Can you work these out from the model? Positions are in its coordinate system, mm. A direction names the side the tool comes from. Coordinates: 2 decimals unless noted, no trailing zeros. Loops run counter-clockwise (first coordinate to the right, second up) from the corner with the lowest first, then second, coordinate; pieces in that order, holes last.
```python
from build123d import *

# Parameters (mm, degrees)
BOSS_EXTRUDE1_DEPTH      = 22
SKETCH1_3_R              = 25
BOSS_EXTRUDE2_DEPTH      = 44
BOSS_EXTRUDE2_DEPTH_BACK = 37


with BuildPart() as part:
    # Sketch1 → Boss-Extrude1 (new body)
    with BuildSketch(Plane.XY):
        Polygon((-177.8, 78.062396106), (177.8, 78.062396106), (101.6, -48.937603894), (-101.6, -48.937603894), align=None)
    extrude(amount=BOSS_EXTRUDE1_DEPTH)

    # Sketch1_3 → Boss-Extrude2 (add, two sides)
    with BuildSketch(Plane.XY) as boss_extrude2_sk:
        with Locations((177.8, 78.062396106)):
            Circle(SKETCH1_3_R)
        with Locations((101.6, -48.937603894)):
            Circle(SKETCH1_3_R)
        with Locations((-101.6, -48.937603894)):
            Circle(SKETCH1_3_R)
        with Locations((-177.8, 78.062396106)):
            Circle(SKETCH1_3_R)
    extrude(amount=BOSS_EXTRUDE2_DEPTH)
    extrude(boss_extrude2_sk.sketch, amount=-BOSS_EXTRUDE2_DEPTH_BACK)


solid = part.part
```
(1) I want a section at D-D on x = -177.8. Write out the boundary of the cut face in (y, z), then the cut area to 3 significant figures.
Check values:
outline: (53.06, -37) - (103.06, -37) - (103.06, 44) - (53.06, 44) - close
area: 4,050 mm2
(2) Which directions (+Z, -Z, +X, -X, +Y, -Y) give clear straight access to the entire face, cutting with the end or side of a thin tool? Please do faces 3 (the flat face through (-178, 78, -37)), 4 (the flat face through (-2, 78.062, 11)).
Check values:
face 3: -Z, +X, -X, +Y, -Y
face 4: +Z, -Z, +Y
(3) If I drill on probe 1 along X at (y, z) = (76, 26.5); probe 2 along X at (y, z) = (78, 40); probe 3 along Y at (x, z) = (-31.5, 14.5), over which ranges is the centre line in solid material (lowest first)?
Check values:
probe 1: x = -202.71 to -152.89, 152.89 to 202.71
probe 2: x = -202.8 to -152.8, 152.8 to 202.8
probe 3: y = -48.94 to 78.06
(4) I want a section at B-B on z = 27.5. Write out the boundary of the cut face in (x, y), then the cut area to 3 significant figures.
Check values:
outline: circle Ø50 at (-177.8, 78.06); circle Ø50 at (-101.6, -48.94); circle Ø50 at (101.6, -48.94); circle Ø50 at (177.8, 78.06)
area: 7,850 mm2
(5) If we mould it in two halves opening along X, with no side actions, what happens to faces 1 (the flat face through (-178, 78, 44)), 2 (the flat face through (1, -48.938, 11))? For each: released by +X, released by -X, zero draft, split by the parting line, or undercut.
Check values:
face 1: zero draft
face 2: undercut
(6) I want a section at C-C on y = 23. Write out the boundary of the cut face in (x, z), then the cut area to 3 significant figures.
Check values:
outline: (-144.76, 0) - (144.76, 0) - (144.76, 22) - (-144.76, 22) - close
area: 6,370 mm2
(7) I want a section at A-A on x = 101.6. Write out the boundary of the cut face in (y, z).
Check values:
outline: (-73.94, -37) - (-23.94, -37) - (-23.94, 0) - (78.06, 0) - (78.06, 22) - (-23.94, 22) - (-23.94, 44) - (-73.94, 44) - close
(8) I'm going to push flat-ended pins straight in: pin 1 (24 mm diameter, centred on x = 11.5, z = 13.5, fed in from -Y); pin 2 (4 mm diameter, centred on x = -50.5, y = -6.5, fed in from +Z); pin 3 (6 mm diameter, centred on y = 15, z = 12, fed in from -X); pin 4 (8 mm diameter, centred on y = -8.5, z = 27.5, fed in from +X). Where does each tip first touch, or does it pass through?
Check values:
pin 1: stops at y = -48.94
pin 2: stops at z = 22
pin 3: stops at x = -141.76
pin 4: passes through
